```python
from build123d import *

# Parameters (mm, degrees)
F3_R     = 5.08
F4_R     = 12.7
F5_DEPTH = 2.54
F6_R     = 12.573
F7_DEPTH = 5.08


with BuildPart() as f2:
    # F0 (on Front) → F2 section 0
    with BuildSketch(Plane.XZ, mode=Mode.PRIVATE) as f2_s0:
        Polygon((-44.901281, 0), (0, -44.901281), (44.901281, 0), (0, 44.901281), align=None)
    loft([f2_s0.sketch, Vertex(0, -20.32, 0)])

    # F3
    f3_edges = [f2.edges().sort_by_distance(p)[0] for p in [
        (22.45064, 0, 22.45064),
        (-22.45064, 0, 22.45064),
        (-22.45064, 0, -22.45064),
        (22.45064, 0, -22.45064),
    ]]
    fillet(f3_edges, radius=F3_R)

    # F4 (on face) → F5 (join)
    with BuildSketch(Plane(origin=(0, 0, 0), x_dir=(-1, 0, 0), z_dir=(0, 1, 0))):
        Circle(F4_R)
    extrude(amount=F5_DEPTH)

    # F6 (on face) → F7 (join)
    with BuildSketch(Plane(origin=(0, 2.54, 0), x_dir=(-1, 0, 0), z_dir=(0, 1, 0))):
        Circle(F6_R)
    extrude(amount=F7_DEPTH)


solid = f2.part
```
Read the model definition and answer for the solid it produces. Units are mm, in the model's axes. A direction names the side the tool comes from. Coordinates: 2 decimals unless noted, no trailing zeros. Loops run counter-clockwise (first coordinate to the right, second up) from the corner with the lowest first, then second, coordinate; pieces in that order, holes last.
(1) A tool of negligible diameter and unlimited length cuts with its end or side. For faces 1 (the face through (-13.45, -3.74, -13.83)), 2 (the face through (-5, 0, 12)), from which of +Z, -Z, +X, -X, +Y, -Y can it reach the whole face along a straight path? Write none if from no direction.
Solution:
face 1: -Z, -X
face 2: +Y
(2) The part is cut by section A-A (y = 1.75). Determine the outline of the cut face in (x, z), and give its area (3 significant figures).
Solution:
outline: circle Ø25.4 at (0, 0)
area: 507 mm2
(3) Flat-ended cylindrical pins translate along their axes: pin 1 Ø12 at (y, z) = (-6, 9) entering from -X; pin 2 Ø1.5 at (x, y) = (-15.5, -3) entering from -Z; pin 3 Ø12 at (x, z) = (20.5, -5.5) entering from -Y. Find the tip coordinate at first contact, or state that the pin passes through.
Solution:
pin 1: stops at x = -24.49
pin 2: stops at z = -12.27
pin 3: stops at y = -12.39
(4) The part is cut by section D-D (y = -18.5). Determine the outline of the cut face in (x, z).
Solution:
outline: (-4.02, 0) - (0, -4.02) - (4.02, 0) - (0, 4.02) - close
(5) Consider line 1 along Y through (x, z) = (-0.5, 3); line 2 along Y through (x, z) = (7, 6); line 3 along X through (y, z) = (-12.25, 13). Determine where each line is inside the solid, lowest interval first.
Solution:
line 1: y = -18.74 to 7.62
line 2: y = -14.44 to 7.62
line 3: x = -4.83 to 4.83
(6) The part is cut by section C-C (y = -6). Determine the outline of the cut face in (x, z), and give its area (3 significant figures).
Solution:
outline: (-27.41, 0) - (0, -27.41) - (27.41, 0) - (0, 27.41) - close
area: 1,500 mm2
(7) The part is cut by section B-B (y = 5.75). Determine the outline of the cut face in (x, z), and give its area (3 significant figures).
Solution:
outline: circle Ø25.15 at (0, 0)
area: 497 mm2
